Could you check a few things on this model? Use its own coordinates, in mm. Face numbers are marked on the shaded views. A direction names the side the tool comes from. Round coordinates to 2 decimals unless told otherwise and drop trailing zeros. Order: outer loops, then holes, each group sorted by start corner. A loop starts at its lowest first (then second) coordinate and runs counter-clockwise, first axis right, second up. Notation, with made-up numbers: M -3,38.25 L 19,38.25 A20 ccw 19,56.25 Z; hole C 58,-2.75 d11. An arc over 180 degrees is marked long. Write each question's results on one line, items separated by ' | '. Start each with the question number.
1. We'd pull the mould along X, two halves only. Please class the marked faces 3, 4 and 5: released by +X, released by -X, zero draft, split by the parting line, or undercut.
2. Suppose I cut it at C-C on x = 3. Write out the boundary of the cut face in (y, z).
3. I'm going to push flat-ended pins straight in: pin 1 (1.5 mm diameter, centred on y = -19.5, z = 12.5, fed in from +X); pin 2 (1 mm diameter, centred on y = -4, z = 18.5, fed in from -X); pin 3 (5.5 mm diameter, centred on x = -151.9, y = 9.59, fed in from -Z). Where does each tip first touch, or does it pass through?
4. Please list where these lines run through material, in increasing order: L1, parallel to Y at x = 5.5, z = 3.25; L2, parallel to X at y = 18, z = 13.75; L3, parallel to X at y = 42, z = 12.25.
5. Suppose I cut it at B-B on x = -50.5. Write out the boundary of the cut face in (y, z).
6. Suppose I cut it at A-A on z = 15.5. Write out the boundary of the cut face in (x, y), and give its area (3 significant figures).
7. For the marked faces 1 and 2, which set-ups out of +Z, -Z, +X, -X, +Y, -Y let a thin tool reach every point of the face, with its end or its side?
from build123d import *

# Parameters (mm, degrees)
EXTRUDE_3_DEPTH     = 30
CUT_EXTRUDE_1_DEPTH = 27.75
SKETCH_5_R          = 1.75
CUT_EXTRUDE_2_DEPTH = 250.931131666
SKETCH_6_R          = 2
CUT_EXTRUDE_3_DEPTH = 251.190943233


with BuildPart() as part:
    # 草图1 → 凸台-拉伸3 (new body)
    with BuildSketch(Plane.XY):
        with BuildLine():
            ThreePointArc((188.956439237, 0), (176.309013441, 23.14413618), (150, 25))
            Line((150, 25), (150, -25))
            ThreePointArc((150, -25), (176.309013441, -23.14413618), (188.956439237, 0))
        make_face()
        with BuildLine():
            Line((150, -25), (150, 25))
            ThreePointArc((150, 25), (133.956439237, 0), (150, -25))
        make_face()
        with BuildLine():
            ThreePointArc((188.956439237, 0), (176.309013441, 23.14413618), (150, 25))
            Line((150, 25), (150, -25))
            ThreePointArc((150, -25), (176.309013441, -23.14413618), (188.956439237, 0))
        make_face()
        with BuildLine():
            Line((150, -25), (150, 25))
            ThreePointArc((150, 25), (133.956439237, 0), (150, -25))
        make_face()
        with BuildLine():
            Line((150, 25), (-150, 25))
            ThreePointArc((-150, 25), (-145.004978875, 12.940952255), (-143.301270189, 0))
            ThreePointArc((-143.301270189, 0), (-145.004978875, -12.940952255), (-150, -25))
            ThreePointArc((-150, -25), (0, -7.455532034), (150, -25))
            ThreePointArc((150, -25), (133.956439237, 0), (150, 25))
        make_face()
        with BuildLine():
            ThreePointArc((-150, 25), (0, 41.260283441), (150, 25))
            Line((150, 25), (-150, 25))
        make_face()
        with BuildLine():
            ThreePointArc((-143.301270189, 0), (-145.004978875, 12.940952255), (-150, 25))
            Line((-150, 25), (-150, -25))
            ThreePointArc((-150, -25), (-145.004978875, -12.940952255), (-143.301270189, 0))
        make_face()
        with BuildLine():
            Line((-150, -25), (-150, 25))
            ThreePointArc((-150, 25), (-243.301270189, 0), (-150, -25))
        make_face()
        with BuildLine():
            ThreePointArc((-143.301270189, 0), (-145.004978875, 12.940952255), (-150, 25))
            Line((-150, 25), (-150, -25))
            ThreePointArc((-150, -25), (-145.004978875, -12.940952255), (-143.301270189, 0))
        make_face()
        with BuildLine():
            Line((-150, -25), (-150, 25))
            ThreePointArc((-150, 25), (-243.301270189, 0), (-150, -25))
        make_face()
    extrude(amount=EXTRUDE_3_DEPTH)

    # 草图3 → 切除-拉伸1 (cut)
    with BuildSketch(Plane(origin=(0, 0, 0), x_dir=(-1, 0, 0), z_dir=(0, 0, -1))):
        with BuildLine():
            ThreePointArc((241.460241998, 2.962420354), (203.950254971, 47.06019149), (151.10937756, 23.40740687))
            Line((151.10937756, 23.40740687), (145.115292459, -2.484763599))
            ThreePointArc((145.115292459, -2.484763599), (182.186192507, -46.952290127), (235.258997062, -23.8246019))
            Line((235.258997062, -23.8246019), (238.35961953, -10.431090773))
            Line((238.35961953, -10.431090773), (241.460241998, 2.962420354))
        make_face()
    extrude(amount=-CUT_EXTRUDE_1_DEPTH, mode=Mode.SUBTRACT)

    # 草图5 → 切除-拉伸2 (cut, through all)
    with BuildSketch(Plane(origin=(0, 0, 27.75), x_dir=(-1, 0, 0), z_dir=(0, 0, -1))):
        with Locations((151.896300525, 9.585326657)):
            Circle(SKETCH_5_R)
        with Locations((170.801384844, 36.055584303)):
            Circle(SKETCH_5_R)
        with Locations((202.886596846, 41.404969664)):
            Circle(SKETCH_5_R)
        with Locations((229.356854492, 22.499885346)):
            Circle(SKETCH_5_R)
        with Locations((234.706239853, -9.585326656)):
            Circle(SKETCH_5_R)
        with Locations((215.801155535, -36.055584303)):
            Circle(SKETCH_5_R)
        with Locations((183.715943533, -41.404969664)):
            Circle(SKETCH_5_R)
        with Locations((157.245685886, -22.499885346)):
            Circle(SKETCH_5_R)
    extrude(amount=-CUT_EXTRUDE_2_DEPTH, mode=Mode.SUBTRACT)

    # 草图6 → 切除-拉伸3 (cut, through all)
    with BuildSketch(Plane.XY.offset(30)):
        with Locations((178.706439237, 0)):
            Circle(SKETCH_6_R)
        with Locations((170.081439237, -14.938938215)):
            Circle(SKETCH_6_R)
        with Locations((152.831439237, -14.938938215)):
            Circle(SKETCH_6_R)
        with Locations((144.206439237, 0)):
            Circle(SKETCH_6_R)
        with Locations((152.831439237, 14.938938215)):
            Circle(SKETCH_6_R)
        with Locations((170.081439237, 14.938938215)):
            Circle(SKETCH_6_R)
    extrude(amount=-CUT_EXTRUDE_3_DEPTH, mode=Mode.SUBTRACT)


solid = part.part
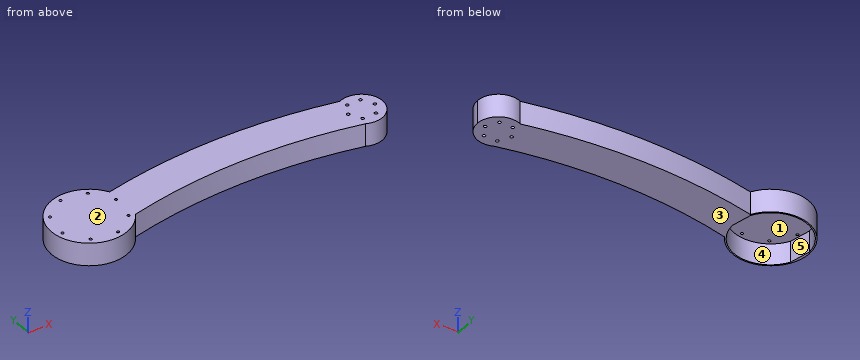
Filled sheet:
1) face 3: zero draft | face 4: undercut | face 5: undercut
2) outline: M -7.46,0 L 41.25,0 L 41.25,30 L -7.46,30 Z
3) pin 1: stops at x = 181.57 | pin 2: stops at x = -243.18 | pin 3: stops at z = 27.75
4) L1: y = -7.48 to 41.24 | L2: x = -239.95 to -238.07, -149.86 to 182.25 | L3: x = -220.43 to -217.05, -169.55 to -166.17
5) outline: M -9.42,0 L 39.44,0 L 39.44,30 L -9.42,30 Z
6) outline: M -150,-25 A650 cw 150,-25 A27.5 ccw long 150,25 A700 ccw -150,25 A50 ccw long Z; hole M -241.46,2.96 L -235.26,-23.82 A48.25 ccw -145.12,-2.48 L -151.11,23.41 A48.25 ccw Z; hole C 144.21,0 d4; hole C 152.83,-14.94 d4; hole C 152.83,14.94 d4; hole C 170.08,-14.94 d4; hole C 170.08,14.94 d4; hole C 178.71,0 d4 | area: 16,800 mm^2
7) face 1: -Z | face 2: +Z, +X, -X, +Y, -Y
